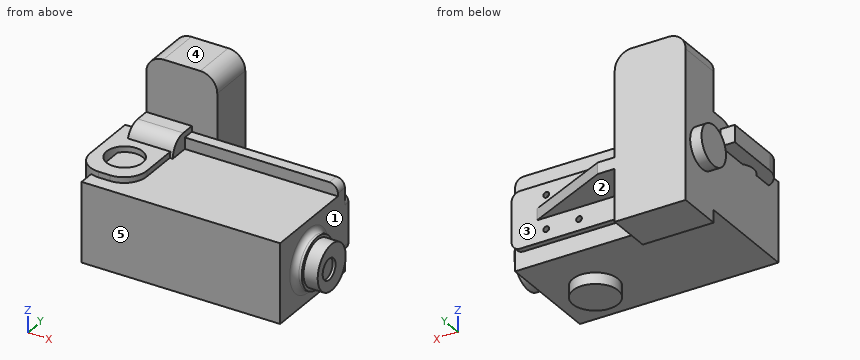
```python
from build123d import *

# Parameters (mm, degrees)
BOSS_EXTRUDE1_DEPTH       = 150
BOSS_EXTRUDE1_DEPTH_BACK  = 100
SKETCH1_W                 = 250
SKETCH1_H                 = 230
SKETCH2_W                 = 200
SKETCH2_H                 = 30
BOSS_EXTRUDE2_DEPTH       = 150
BOSS_EXTRUDE3_DEPTH       = 120
BOSS_EXTRUDE3_DEPTH_BACK  = 20
SKETCH4_W                 = 350
SKETCH4_H                 = 165
RIB1_REACH                = 447.477
SKETCH5_WALL_W            = 1072.6047598
SKETCH5_WALL_H            = 250
SKETCH6_R                 = 45
BOSS_EXTRUDE4_DEPTH       = 15
SKETCH7_R                 = 40
BOSS_EXTRUDE5_DEPTH       = 20
SKETCH8_W                 = 100
SKETCH8_H                 = 100
SKETCH10_W                = 20
SKETCH10_H                = 100
BOSS_EXTRUDE6_DEPTH       = 150
RIB2_REACH                = 449.985
SKETCH12_WALL_W           = 999.204922194
SKETCH12_WALL_H           = 20
SKETCH13_R                = 32
CUT_EXTRUDE1_DEPTH        = 10
FILLET1_R                 = 50
FILLET2_R                 = 30
FILLET3_R                 = 15
FILLET4_R                 = 15
SKETCH14_R                = 40
SKETCH14_R_2              = 18.360426304
BOSS_EXTRUDE7_DEPTH       = 5
FILLET6_R                 = 10
SKETCH15_W                = 250
SKETCH15_H                = 230
SKETCH15_W_2              = 170
SKETCH15_H_2              = 165.671954638
CUT_EXTRUDE2_DEPTH        = 40
SKETCH16_R                = 50
SKETCH16_R_2              = 30
BOSS_EXTRUDE8_DEPTH       = 30
SKETCH16_2_R              = 30
BOSS_EXTRUDE9_DEPTH       = 50
SKETCH17_W                = 787.442297404
SKETCH17_H                = 468.570764298
CUT_EXTRUDE3_DEPTH        = 459.262102583
SKETCH18_W                = 754.820557273
SKETCH18_H                = 297.051261894
CUT_EXTRUDE4_DEPTH        = 391.736484091
BOSS_EXTRUDE10_DEPTH      = 30
BOSS_EXTRUDE11_DEPTH      = 20
BOSS_EXTRUDE12_DEPTH      = 100
BOSS_EXTRUDE12_DEPTH_BACK = 192
SKETCH23_W                = 125
SKETCH23_H                = 80
SKETCH26_W                = 38.43559463
SKETCH26_H                = 130.536564267
CUT_EXTRUDE8_DEPTH        = 196
SKETCH27_W                = 225
SKETCH27_H                = 100
BOSS_EXTRUDE14_DEPTH      = 10
BOSS_EXTRUDE15_DEPTH      = 10
BOSS_EXTRUDE15_DEPTH_BACK = 10
SKETCH29_R                = 35
BOSS_EXTRUDE16_DEPTH      = 20
FILLET7_R                 = 15
FILLET9_R                 = 15
SKETCH33_R                = 40
BOSS_EXTRUDE17_DEPTH      = 20
SKETCH31_R                = 5
CUT_EXTRUDE10_DEPTH       = 10
BOSS_EXTRUDE18_DEPTH      = 10
BOSS_EXTRUDE18_DEPTH_BACK = 20
SKETCH20_R                = 32
FILLET10_R                = 30
SCALE1_SCALE              = 0.6


with BuildPart() as part:
    # Sketch1 → Boss-Extrude1 (new, two sides: drawn at the far end of the back side and taken through both)
    with BuildSketch(Plane(origin=(0, 0, 0), x_dir=(1, 0, 0), z_dir=(0, 1, 0)).offset(-BOSS_EXTRUDE1_DEPTH_BACK)):
        Rectangle(SKETCH1_W, SKETCH1_H)
    extrude(amount=BOSS_EXTRUDE1_DEPTH + BOSS_EXTRUDE1_DEPTH_BACK)

    # Sketch2 → Boss-Extrude2 (add)
    with BuildSketch(Plane(origin=(125, 0, 0), x_dir=(0, 0, -1), z_dir=(1, 0, 0))):
        with Locations((0, -15)):
            Rectangle(SKETCH2_W, SKETCH2_H)
    extrude(amount=BOSS_EXTRUDE2_DEPTH)

    # Sketch4 → Boss-Extrude3 (add, two sides: drawn at the far end of the back side and taken through both)
    with BuildSketch(Plane(origin=(0, 0, -115), x_dir=(-1, 0, 0), z_dir=(0, 0, -1)).offset(-BOSS_EXTRUDE3_DEPTH_BACK)):
        with Locations((-50, 177.5)):
            Rectangle(SKETCH4_W, SKETCH4_H)
    extrude(amount=BOSS_EXTRUDE3_DEPTH + BOSS_EXTRUDE3_DEPTH_BACK)

    # Sketch5 wall → Rib1 (add, up to next)
    with BuildSketch(Plane(origin=(0, 205, -23.982044646), x_dir=(0, 0.612300963241, -0.790624772199), z_dir=(0, 0.790624772199, 0.612300963241)), mode=Mode.PRIVATE) as rib1_sk1:
        Rectangle(SKETCH5_WALL_W, SKETCH5_WALL_H)
    rib1_tool1 = extrude(rib1_sk1.sketch, amount=-RIB1_REACH, mode=Mode.PRIVATE) - part.part
    add(rib1_tool1.solids().sort_by_distance((0, 205, -23.982044646))[0])

    # Sketch6 → Boss-Extrude4 (add)
    with BuildSketch(Plane(origin=(225, 0, 0), x_dir=(0, 0, -1), z_dir=(1, 0, 0))):
        with Locations(Location((165, 177.5, 0), (0, 0, 90))):
            Circle(SKETCH6_R)
    extrude(amount=BOSS_EXTRUDE4_DEPTH)

    # Sketch7 → Boss-Extrude5 (add)
    with BuildSketch(Plane(origin=(240, 0, 0), x_dir=(0, 0, -1), z_dir=(1, 0, 0))):
        with Locations(Location((165, 177.5, 0), (0, 0, 90))):
            Circle(SKETCH7_R)
    extrude(amount=BOSS_EXTRUDE5_DEPTH)

    # Sweep1: sweep along a path in Sketch9
    with BuildLine(Plane(origin=(0, 0, 0), x_dir=(0, 0, -1), z_dir=(1, 0, 0))) as sweep1_path:
        ThreePointArc((23.982044646, 205), (3.428361586, 247.544867247), (-5.288861265, 293.983317287))
    # Sketch8 → Sweep1 (sweep)
    with BuildSketch(Plane(origin=(0, 116.533228497, 90.24939588), x_dir=(1, 0, 0), z_dir=(0, 0.7906247721978943, 0.6123009632419566))):
        with Locations((0, 144.482496049)):
            Rectangle(SKETCH8_W, SKETCH8_H)
    sweep(path=sweep1_path.line)

    # Sketch10 → Boss-Extrude6 (add)
    with BuildSketch(Plane(origin=(125, 0, 0), x_dir=(0, 0, -1), z_dir=(1, 0, 0))):
        with Locations((85, 164.273096985)):
            Rectangle(SKETCH10_W, SKETCH10_H)
    extrude(amount=BOSS_EXTRUDE6_DEPTH)

    # Sketch12 wall → Rib2 (add, up to next)
    with BuildSketch(Plane(origin=(160.792179202, 164.273096985, -35.792179202), x_dir=(0.707106781187, 0, -0.707106781187), z_dir=(0.707106781187, 0, 0.707106781187)), mode=Mode.PRIVATE) as rib2_sk1:
        Rectangle(SKETCH12_WALL_W, SKETCH12_WALL_H)
    rib2_tool1 = extrude(rib2_sk1.sketch, amount=-RIB2_REACH, mode=Mode.PRIVATE) - part.part
    add(rib2_tool1.solids().sort_by_distance((160.792179202, 164.273096985, -35.792179202))[0])

    # Sketch13 → Cut-Extrude1 (cut)
    with BuildSketch(Plane.XZ.offset(30)):
        with Locations(Location((218.869669038, 0, 0), (0, 0, 270))):
            Circle(SKETCH13_R)
    extrude(amount=-CUT_EXTRUDE1_DEPTH, mode=Mode.SUBTRACT)

    # Fillet1
    fillet1_edges = [part.edges().sort_by_distance(p)[0] for p in [
        (275, -15, 100),
        (275, -15, -100),
    ]]
    fillet(fillet1_edges, radius=FILLET1_R)

    # Fillet2
    fillet2_edges = [part.edges().sort_by_distance(p)[0] for p in [
        (125, 95, -105),
    ]]
    fillet(fillet2_edges, radius=FILLET2_R)

    # Fillet3
    fillet3_edges = [part.edges().sort_by_distance(p)[0] for p in [
        (125, 214.273096985, -85),
        (125, 114.273096985, -85),
    ]]
    fillet(fillet3_edges, radius=FILLET3_R)

    # Fillet4
    fillet4_edges = [part.edges().sort_by_distance(p)[0] for p in [
        (50, 205, -23.982044646),
        (0, 235.615048162, -63.513283256),
        (-50, 205, -23.982044646),
        (0, 174.384951838, 15.549193964),
    ]]
    fillet(fillet4_edges, radius=FILLET4_R)

    # Sketch14 → Boss-Extrude7 (add)
    with BuildSketch(Plane(origin=(260, 0, 0), x_dir=(0, 0, -1), z_dir=(1, 0, 0))):
        with Locations(Location((165, 177.5, 0), (0, 0, 90))):
            Circle(SKETCH14_R)
        with Locations(Location((165, 170, 0), (0, 0, 90))):
            Circle(SKETCH14_R_2, mode=Mode.SUBTRACT)
    extrude(amount=BOSS_EXTRUDE7_DEPTH)

    # Fillet6
    fillet6_edges = [part.edges().sort_by_distance(p)[0] for p in [
        (225, 132.5, -165),
    ]]
    fillet(fillet6_edges, radius=FILLET6_R)

    # Sketch15 → Cut-Extrude2 (cut)
    with BuildSketch(Plane.XZ.offset(100)):
        Rectangle(SKETCH15_W, SKETCH15_H)
        Rectangle(SKETCH15_W_2, SKETCH15_H_2, mode=Mode.SUBTRACT)
    extrude(amount=-CUT_EXTRUDE2_DEPTH, mode=Mode.SUBTRACT)

    # Sketch16 → Boss-Extrude8 (add)
    with BuildSketch(Plane.ZY.offset(125)):
        with Locations((0, 30)):
            Circle(SKETCH16_R)
        with Locations((0, 30)):
            Circle(SKETCH16_R_2, mode=Mode.SUBTRACT)
    extrude(amount=BOSS_EXTRUDE8_DEPTH)

    # Sketch16<2> → Boss-Extrude9 (add)
    with BuildSketch(Plane.ZY.offset(125)):
        with Locations((0, 30)):
            Circle(SKETCH16_2_R)
    extrude(amount=BOSS_EXTRUDE9_DEPTH)

    # Sketch17 → Cut-Extrude3 (cut, through all)
    with BuildSketch(Plane.XY.offset(-95)):
        with Locations((43.842387257, 99.928182048)):
            Rectangle(SKETCH17_W, SKETCH17_H)
    extrude(amount=CUT_EXTRUDE3_DEPTH, mode=Mode.SUBTRACT)

    # Sketch18 → Cut-Extrude4 (cut, through all)
    with BuildSketch(Plane.XZ.offset(-95)):
        with Locations((103.1212944, -159.735098903)):
            Rectangle(SKETCH18_W, SKETCH18_H)
    extrude(amount=CUT_EXTRUDE4_DEPTH, mode=Mode.SUBTRACT)

    # Sketch19 → Boss-Extrude10 (add)
    with BuildSketch(Plane(origin=(0, 0, -95), x_dir=(-1, 0, 0), z_dir=(0, 0, -1))):
        Polygon((125, 260), (44.807978096, 260), (44.807978096, 161.220017504), (100, 95), (125, 177.5), align=None)
    extrude(amount=-BOSS_EXTRUDE10_DEPTH)

    # Sketch22 → Boss-Extrude11 (add)
    with BuildSketch(Plane(origin=(0, 260, 0), x_dir=(1, 0, 0), z_dir=(0, 1, 0))):
        Polygon((225, 95), (225, 75), (-44.807978096, 75), (-44.807978096, 65), (-125, 65), (-125, 235), (225, 235), align=None)
    extrude(amount=BOSS_EXTRUDE11_DEPTH)

    # Sketch23 → Boss-Extrude12 (add, two sides: drawn at the far end of the back side and taken through both)
    with BuildSketch(Plane.XY.offset(-65).offset(-BOSS_EXTRUDE12_DEPTH_BACK)):
        with Locations((-62.5, 320)):
            Rectangle(SKETCH23_W, SKETCH23_H)
    extrude(amount=BOSS_EXTRUDE12_DEPTH + BOSS_EXTRUDE12_DEPTH_BACK)

    # Sketch26 → Cut-Extrude8 (cut)
    with BuildSketch(Plane(origin=(-44.807978096, 0, 0), x_dir=(0, 0, -1), z_dir=(1, 0, 0))):
        with Locations((75.782202685, 160.268282134)):
            Rectangle(SKETCH26_W, SKETCH26_H)
    extrude(amount=-CUT_EXTRUDE8_DEPTH, mode=Mode.SUBTRACT)

    # Sketch27 → Boss-Extrude14 (add)
    with BuildSketch(Plane(origin=(0, 280, 0), x_dir=(1, 0, 0), z_dir=(0, 1, 0))):
        with Locations((112.5, 155)):
            Rectangle(SKETCH27_W, SKETCH27_H)
    extrude(amount=BOSS_EXTRUDE14_DEPTH)

    # Sketch28 → Boss-Extrude15 (add, two sides: drawn at the far end of the back side and taken through both)
    with BuildSketch(Plane.XY.offset(-155).offset(-BOSS_EXTRUDE15_DEPTH_BACK)):
        Polygon((0, 360), (0, 290), (180.556109721, 290), (30, 360), align=None)
    extrude(amount=BOSS_EXTRUDE15_DEPTH + BOSS_EXTRUDE15_DEPTH_BACK)

    # Sketch29 → Boss-Extrude16 (add)
    with BuildSketch(Plane.ZY.offset(125)):
        with Locations((-145, 312.056134744)):
            Circle(SKETCH29_R)
    extrude(amount=BOSS_EXTRUDE16_DEPTH)

    # Fillet7
    fillet7_edges = [part.edges().sort_by_distance(p)[0] for p in [
        (225, 270, -75),
    ]]
    fillet(fillet7_edges, radius=FILLET7_R)

    # Fillet9
    fillet9_edges = [part.edges().sort_by_distance(p)[0] for p in [
        (225, 285, -205),
        (225, 285, -105),
    ]]
    fillet(fillet9_edges, radius=FILLET9_R)

    # Sketch33 → Boss-Extrude17 (add)
    with BuildSketch(Plane(origin=(0, 0, -235), x_dir=(-1, 0, 0), z_dir=(0, 0, -1))):
        with Locations(Location((-145, 180, 0), (0, 0, 180))):
            Circle(SKETCH33_R)
    extrude(amount=BOSS_EXTRUDE17_DEPTH)

    # Sketch31 → Cut-Extrude10 (cut)
    with BuildSketch(Plane(origin=(0, 290, 0), x_dir=(1, 0, 0), z_dir=(0, 1, 0))):
        with Locations(Location((106.129760479, 125.68527506, 0), (0, 0, 180))):
            Circle(SKETCH31_R)
        with Locations(Location((163.912196034, 125.68527506, 0), (0, 0, 180))):
            Circle(SKETCH31_R)
        with Locations((230.176456992, 125.68527506)):
            Circle(SKETCH31_R)
        with Locations(Location((163.912196034, 185.323109922, 0), (0, 0, 180))):
            Circle(SKETCH31_R)
        with Locations(Location((106.129760479, 185.323109922, 0), (0, 0, 180))):
            Circle(SKETCH31_R)
        with Locations((230.176456992, 185.323109922)):
            Circle(SKETCH31_R)
    extrude(amount=-CUT_EXTRUDE10_DEPTH, mode=Mode.SUBTRACT)

    # Sketch20 → Boss-Extrude18 (add, two sides: drawn at the far end of the back side and taken through both)
    with BuildSketch(Plane.XY.offset(-95).offset(-BOSS_EXTRUDE18_DEPTH_BACK)):
        with BuildLine():
            Line((-50, 260), (-50, 159.605646018))
            ThreePointArc((-50, 159.605646018), (-61.715728753, 131.321374771), (-90, 119.605646018))
            Line((-90, 119.605646018), (-110, 119.605646018))
            ThreePointArc((-110, 119.605646018), (-138.284271247, 131.321374771), (-150, 159.605646018))
            Line((-150, 159.605646018), (-150, 260))
            Line((-150, 260), (-50, 260))
        make_face()
        with Locations((-100, 177.5)):
            Circle(SKETCH20_R, mode=Mode.SUBTRACT)
    extrude(amount=BOSS_EXTRUDE18_DEPTH + BOSS_EXTRUDE18_DEPTH_BACK)

    # Fillet10
    fillet10_edges = [part.edges().sort_by_distance(p)[0] for p in [
        (-84.903989048, 225.536564267, -65),
        (-125, 320, 35),
        (0, 320, 35),
    ]]
    fillet(fillet10_edges, radius=FILLET10_R - 0.0001)  # a hair under: the kernel refuses the full size


with BuildPart() as part_1:
    # Scale1: scaled about (26.616775413, 221.668719116, -151.512951555)
    add(part.part.scale(SCALE1_SCALE).moved(Location((10.646710165, 88.667487646, -60.605180622))))


solid = part_1.part
```
The model under review builds one solid part; all positions refer to its coordinate system, in mm. Face numbers are marked on the shaded views. A direction names the side the tool comes from. Round coordinates to 2 decimals unless told otherwise and drop trailing zeros. Loops run counter-clockwise (first coordinate to the right, second up) from the corner with the lowest first, then second, coordinate; pieces in that order, holes last.
1) Wall thickness on line 1 along Y through (x, z) = (19, -161.5); line 2 along X through (y, z) = (281.5, -64); line 3 along Z through (x, y) = (111.5, 235): over which ranges is each line inside the solid? List them lowest first.
Values follow:
line 1: y = 145.67 to 262.67
line 2: x = -64.35 to 10.65
line 3: z = -201.61 to -117.61
2) Consider section B-B on y = 231. State the section outline as (x, z) points, then the cut area to 3 significant figures.
Values follow:
outline: (-79.35, -129.61) - (-64.35, -129.61) - (-64.35, -201.61) - (145.65, -201.61) - (145.65, -117.61) - (-16.24, -117.61) - (-16.24, -103.35) - (-64.35, -103.35) - (-64.35, -111.61) - (-79.35, -111.61) - close
area: 18,600 mm2
3) Tool access review of the marked faces 1, 2, 3, 4 and 5: name each direction out of +Z, -Z, +X, -X, +Y, -Y from which nothing blocks a thin tool from reaching the whole face with its end or side.
Values follow:
face 1: +X
face 2: -Z, +X, +Y
face 3: +X, +Y
face 4: +Z, +X, -X, +Y, -Y
face 5: +Z, -Z, +X, -X, -Y
4) Consider section D-D on x = -39.5. State the section outline as (y, z) points.
Values follow:
outline: (145.67, -201.61) - (256.67, -201.61) - (256.67, -214.81) - (304.67, -214.81) - (304.67, -39.61) - (256.67, -39.61) - (256.67, -99.61) - (241.99, -99.61) arc R18 ccw to (225.02, -111.61) - (211.65, -111.61) - (211.65, -117.61) - (178.69, -117.61) - (178.69, -111.61) - (160.74, -111.61) - (160.74, -117.61) - (145.67, -117.61) - close
5) Consider section C-C on z = -70. State the section outline as (x, y) points, then the cut area to 3 significant figures.
Values follow:
outline: (-64.35, 256.67) - (10.65, 256.67) - (10.65, 304.67) - (-64.35, 304.67) - close
area: 3,600 mm2
6) Clearance check with flat-ended pins moving along their axes: P1, Ø5, axis at x = -52.5, z = -113.5, coming from the -Y side; P2, Ø3, axis at x = 109, z = -135.5, coming from the +Y side; P3, Ø12, axis at x = 13, z = -77.5, coming from the -Y side. State where each tip first meets the part, or that it passes through.
Values follow:
P1: stops at y = 160.43
P2: stops at y = 256.67
P3: stops at y = 256.67
7) Consider section A-A on x = 65. State the section outline as (y, z) points.
Values follow:
outline: (145.67, -201.61) - (256.67, -201.61) - (256.67, -183.61) - (262.67, -183.61) - (262.67, -159.61) - (287.77, -159.61) - (287.77, -147.61) - (262.67, -147.61) - (262.67, -123.61) - (256.67, -123.61) - (256.67, -105.61) - (244.67, -105.61) - (244.67, -117.61) - (145.67, -117.61) - close
